Autodesk Inventor part; units mm, degrees
ref_plane "rot_XY" through (0, 6.6675, 0) normal (0, 0, 1) x (1, 0, 0)
ref_plane "rot_YZ" through (0, 6.6675, 0) normal (1, 0, 0) x (0, 1, 0)
ref_plane "rot_ZX" through (0, 6.6675, 0) normal (0, 1, 0) x (0, 0, 1)
sketch "Sketch_2" plane through (0, -0.254, 0) normal (0, 1, 0) x (1, 0, 0)
  line L0 (-6.5024, -3.9497) -> (-6.0389, -3.9497)
  line L1 (-6.0389, -3.9497) -> (-6.0389, -3.4862)
  line L2 (-6.0389, -3.4862) -> (-3.2509, -3.4862)
  line L3 (-3.2509, -3.4862) -> (-3.0348, -3.0226)
  line L4 (-3.0348, -3.0226) -> (-2.0452, -3.0226)
  line L5 (-2.0452, -3.0226) -> (-1.8291, -3.4862)
  line L6 (-1.8291, -3.4862) -> (1.8291, -3.4862)
  line L7 (1.8291, -3.4862) -> (2.0452, -3.0226)
  line L8 (2.0452, -3.0226) -> (3.0348, -3.0226)
  line L9 (3.0348, -3.0226) -> (3.2509, -3.4862)
  line L10 (3.2509, -3.4862) -> (6.0389, -3.4862)
  line L11 (6.0389, -3.4862) -> (6.0389, -3.9497)
  line L12 (6.0389, -3.9497) -> (6.5024, -3.9497)
  line L13 (6.5024, -3.9497) -> (6.5024, 3.9497)
  line L14 (6.5024, 3.9497) -> (6.0389, 3.9497)
  line L15 (6.0389, 3.9497) -> (6.0389, 3.4862)
  line L16 (6.0389, 3.4862) -> (3.2509, 3.4862)
  line L17 (3.2509, 3.4862) -> (3.0348, 3.0226)
  line L18 (3.0348, 3.0226) -> (2.0452, 3.0226)
  line L19 (2.0452, 3.0226) -> (1.8291, 3.4862)
  line L20 (1.8291, 3.4862) -> (-1.8291, 3.4862)
  line L21 (-1.8291, 3.4862) -> (-2.0452, 3.0226)
  line L22 (-2.0452, 3.0226) -> (-3.0348, 3.0226)
  line L23 (-3.0348, 3.0226) -> (-3.2509, 3.4862)
  line L24 (-3.2509, 3.4862) -> (-6.0389, 3.4862)
  line L25 (-6.0389, 3.4862) -> (-6.0389, 3.9497)
  line L26 (-6.0389, 3.9497) -> (-6.5024, 3.9497)
  line L27 (-6.5024, 3.9497) -> (-6.5024, -3.9497)
extrude "Extrusion1" add sketch "Sketch_2" against normal blind 9.8476
sketch "Sketch_8" plane through (0, -9.5936, 0) normal (0, 1, 0) x (1, 0, 0)
  line L0 (-5.08, -0.889) -> (-4.318, -0.889)
  line L1 (-4.318, -0.889) -> (-4.318, 0.889)
  line L2 (-4.318, 0.889) -> (-5.08, 0.889)
  line L3 (-5.08, 0.889) -> (-5.08, -0.889)
extrude "Extrusion2" cut sketch "Sketch_8" against normal blind 25.4
sketch "Sketch_5" plane through (0, -9.5936, 0) normal (0, 1, 0) x (1, 0, 0)
  line L0 (-0.381, -0.889) -> (0.381, -0.889)
  line L1 (0.381, -0.889) -> (0.381, 0.889)
  line L2 (0.381, 0.889) -> (-0.381, 0.889)
  line L3 (-0.381, 0.889) -> (-0.381, -0.889)
extrude "Extrusion3" cut sketch "Sketch_5" against normal blind 25.4
sketch "Sketch_9" plane through (0, -9.5936, 0) normal (0, 1, 0) x (1, 0, 0)
  line L0 (4.318, -0.889) -> (5.08, -0.889)
  line L1 (5.08, -0.889) -> (5.08, 0.889)
  line L2 (5.08, 0.889) -> (4.318, 0.889)
  line L3 (4.318, 0.889) -> (4.318, -0.889)
extrude "Extrusion4" cut sketch "Sketch_9" against normal blind 25.4
sketch "Sketch_19" plane through (0, -0.254, 0) normal (0, 1, 0) x (1, 0, 0)
  line L0 (-6.5024, -3.9497) -> (-6.0389, -3.9497)
  line L1 (-6.0389, -3.9497) -> (-6.0389, -3.4862)
  line L2 (-6.0389, -3.4862) -> (-3.2509, -3.4862)
  line L3 (-3.2509, -3.4862) -> (-3.0348, -3.0226)
  line L4 (-3.0348, -3.0226) -> (-2.0452, -3.0226)
  line L5 (-2.0452, -3.0226) -> (-1.8291, -3.4862)
  line L6 (-1.8291, -3.4862) -> (1.8291, -3.4862)
  line L7 (1.8291, -3.4862) -> (2.0452, -3.0226)
  line L8 (2.0452, -3.0226) -> (3.0348, -3.0226)
  line L9 (3.0348, -3.0226) -> (3.2509, -3.4862)
  line L10 (3.2509, -3.4862) -> (6.0389, -3.4862)
  line L11 (6.0389, -3.4862) -> (6.0389, -3.9497)
  line L12 (6.0389, -3.9497) -> (6.5024, -3.9497)
  line L13 (6.5024, -3.9497) -> (6.5024, 3.9497)
  line L14 (6.5024, 3.9497) -> (6.0389, 3.9497)
  line L15 (6.0389, 3.9497) -> (6.0389, 3.4862)
  line L16 (6.0389, 3.4862) -> (3.2509, 3.4862)
  line L17 (3.2509, 3.4862) -> (3.0348, 3.0226)
  line L18 (3.0348, 3.0226) -> (2.0452, 3.0226)
  line L19 (2.0452, 3.0226) -> (1.8291, 3.4862)
  line L20 (1.8291, 3.4862) -> (-1.8291, 3.4862)
  line L21 (-1.8291, 3.4862) -> (-2.0452, 3.0226)
  line L22 (-2.0452, 3.0226) -> (-3.0348, 3.0226)
  line L23 (-3.0348, 3.0226) -> (-3.2509, 3.4862)
  line L24 (-3.2509, 3.4862) -> (-6.0389, 3.4862)
  line L25 (-6.0389, 3.4862) -> (-6.0389, 3.9497)
  line L26 (-6.0389, 3.9497) -> (-6.5024, 3.9497)
  line L27 (-6.5024, 3.9497) -> (-6.5024, -3.9497)
extrude "Extrusion5" cut sketch "Sketch_19" against normal blind 0.254
ref_plane "rot_XY" through (0, 6.6675, 0) normal (0, 0, 1) x (1, 0, 0)
ref_plane "rot_YZ" through (0, 6.6675, 0) normal (1, 0, 0) x (0, 1, 0)
ref_plane "rot_ZX" through (0, 6.6675, 0) normal (0, 1, 0) x (0, 0, 1)
ref_plane "to_cover_XY" through (0, -0.254, 0) normal (0, 1, 0) x (1, 0, 0)
ref_plane "to_cover_YZ" through (0, -0.254, 0) normal (1, 0, 0) x (0, 0, -1)
ref_plane "to_cover_ZX" through (0, -0.254, 0) normal (0, 0, -1) x (0, 1, 0)
ref_plane "to_terminals_XY" through (0, -9.5936, 0) normal (0, -1, 0) x (1, 0, 0)
ref_plane "to_terminals_YZ" through (0, -9.5936, 0) normal (1, 0, 0) x (0, 0, 1)
ref_plane "to_terminals_ZX" through (0, -9.5936, 0) normal (0, 0, 1) x (0, -1, 0)
properties part number "M20_ang1230TX-switch"
Verification items for the finished model (mm, model axes). A direction names the side the tool comes from. Give positions to 0.01 mm unless a question says otherwise; leave off trailing zeros. Order: outer loops, then holes, each group sorted by start corner. A loop starts at its lowest first (then second) coordinate and runs counter-clockwise, first axis right, second up. Notation, with made-up numbers: M -29,10 L 20,10 A29 ccw 20,30 Z; hole C 46.5,-25.75 d5. An arc over 180 degrees is marked long. Use one line per item in the form item = value. Start each with the question number.
Q1. Section check B-B (x = -4.75). Enter the section's corners in (y, z), then the cut area to 3 significant figures.
Q2. Mould release check, pull along X, two halves, no side actions. Record for faces 1 (the flat face through (-2.5, -5.2, 3.023)), 2 (the flat face through (-6.502, -5, 0)), 3 (the flat face through (6.502, -5, 0)): +X half, -X half, draft (parallel to the pull), parting line (faces both ways), or undercut.
Q3. Section check C-C (x = 3.5). Enter the section's corners in (y, z), then the cut area to 3 significant figures.
Q4. Go/stop test with flat-tipped pins: pin 1 Ø1.8 at (x, y) = (0.5, -5) entering from -Z; pin 2 Ø0.5 at (x, y) = (2.5, -7) entering from -Z; pin 3 Ø1.4 at (x, y) = (-5.5, -4.5) entering from -Z; pin 4 Ø1.4 at (x, y) = (4, -7) entering from +Z. Record where each tip stops, or that it passes through.
Q5. Access from +Z, -Z, +X, -X, +Y, -Y to the whole of each face (thin tool, end or side, straight path). Record for faces 4 (the flat face through (-2.5, -5.2, -3.023)), 5 (the flat face through (0, -5, 3.486)), 6 (the flat face through (0, -0.508, 0)).
Q6. Scan lines: line 1 along Z through (x, y) = (4.5, -3.75); line 2 along Z through (x, y) = (2.25, -6.5). Record each from-to range of solid material in increasing order. Write a range as [from, to].
Q7. Section check A-A (y = -5). Enter the section's corners in (x, z), then the cut area to 3 significant figures.
Evaluation:
q1.outline = M -10.1,-3.49 L -0.51,-3.49 L -0.51,3.49 L -10.1,3.49 L -10.1,0.89 L -9.59,0.89 L -9.59,-0.89 L -10.1,-0.89 Z
q1.area = 66.0 mm2
q2.face_1 = undercut
q2.face_2 = -X half
q2.face_3 = +X half
q3.outline = M -10.1,-3.49 L -0.51,-3.49 L -0.51,3.49 L -10.1,3.49 Z
q3.area = 66.9 mm2
q4.pin_1 = -3.49
q4.pin_2 = -3.02
q4.pin_3 = -3.95
q4.pin_4 = 3.49
q5.face_4 = -Z, +Y, -Y
q5.face_5 = +Z, +Y, -Y
q5.face_6 = +Z, -Z, +X, -X, +Y
q6.line_1 = [-3.49, 3.49]
q6.line_2 = [-3.02, 3.02]
q7.outline = M -6.5,-3.95 L -6.04,-3.95 L -6.04,-3.49 L -3.25,-3.49 L -3.03,-3.02 L -2.05,-3.02 L -1.83,-3.49 L 1.83,-3.49 L 2.05,-3.02 L 3.03,-3.02 L 3.25,-3.49 L 6.04,-3.49 L 6.04,-3.95 L 6.5,-3.95 L 6.5,3.95 L 6.04,3.95 L 6.04,3.49 L 3.25,3.49 L 3.03,3.02 L 2.05,3.02 L 1.83,3.49 L -1.83,3.49 L -2.05,3.02 L -3.03,3.02 L -3.25,3.49 L -6.04,3.49 L -6.04,3.95 L -6.5,3.95 Z
q7.area = 89.3 mm2
